The model under review builds one solid part; all positions refer to its coordinate system, in mm. Coordinates: 2 decimals unless noted, no trailing zeros. Loops run counter-clockwise (first coordinate to the right, second up) from the corner with the lowest first, then second, coordinate; pieces in that order, holes last. Notation, with made-up numbers: (15.5, 80.5) - (71.5, 80.5) arc R31 cw to (71.5, 118.5) - close; hole circle Ø1 at (16.5, -28.75). An arc over 180 degrees is marked (long way). Answer in a Markdown table with one row per item. Add a question column.
(1) We need section B-B on z = -37.5. Write out the cut boundary in (x, y), plus the area to 3 significant figures.
(2) We need section D-D on z = 7. Write out the cut boundary in (x, y), plus the area to 3 significant figures.
(3) We need section A-A on y = 5.5. Write out the cut boundary in (x, z), plus the area to 3 significant figures.
(4) We need section C-C on x = 8. Write out the cut boundary in (y, z), plus the area to 3 significant figures.
(5) For line 1 along X through (y, z) = (1.3, 39.5); line 2 along Y through (x, z) = (-46, 37.5); line 3 along X through (y, z) = (10.5, 38), list the stretches that pass through material, from the lowest coordinate up.
(6) For P1, Ø1, axis at x = -46, y = 7, coming from the -Z side; P2, Ø1.6, axis at x = -46.5, y = 6, coming from the +Z side; P3, Ø2, axis at y = 1, z = 0, coming from the -X side; P4, Ø4, axis at x = 27, y = 5.5, coming from the +Z side, all flat-tipped, find the tip position at first contact; note any pin that passes through.
from build123d import *

# Parameters (mm, degrees)
SKETCH1_W           = 95
SKETCH1_H           = 95
BOSS_EXTRUDE1_DEPTH = 2
SKETCH2_W           = 2
SKETCH2_H           = 6
BOSS_EXTRUDE2_DEPTH = 6
SKETCH3_R           = 3
BOSS_EXTRUDE3_DEPTH = 2
SKETCH6_R           = 3
BOSS_EXTRUDE5_DEPTH = 2
SKETCH8_R           = 1.3
CUT_EXTRUDE2_DEPTH  = 96
FILLET1_R           = 2
SKETCH10_W          = 25
SKETCH10_H          = 4
CUT_EXTRUDE3_DEPTH  = 5
SKETCH11_R          = 2.5
CUT_EXTRUDE4_DEPTH  = 2


with BuildPart() as part:
    # Sketch1 → Boss-Extrude1 (new body)
    with BuildSketch(Plane(origin=(0, 0, 0), x_dir=(1, 0, 0), z_dir=(0, 1, 0))):
        Rectangle(SKETCH1_W, SKETCH1_H)
    extrude(amount=BOSS_EXTRUDE1_DEPTH)

    # Sketch2 → Boss-Extrude2 (add)
    with BuildSketch(Plane(origin=(0, 2, 0), x_dir=(1, 0, 0), z_dir=(0, 1, 0))):
        with Locations((-46.5, -37.5)):
            Rectangle(SKETCH2_W, SKETCH2_H)
        with Locations((-46.5, 37.5)):
            Rectangle(SKETCH2_W, SKETCH2_H)
        with Locations((46.5, -37.5)):
            Rectangle(SKETCH2_W, SKETCH2_H)
        with Locations((46.5, 37.5)):
            Rectangle(SKETCH2_W, SKETCH2_H)
    extrude(amount=BOSS_EXTRUDE2_DEPTH)

    # Sketch3 → Boss-Extrude3 (add)
    with BuildSketch(Plane(origin=(-45.5, 0, 0), x_dir=(0, 0, -1), z_dir=(1, 0, 0))):
        with Locations((-37.5, 8)):
            Circle(SKETCH3_R)
        with Locations((37.5, 8)):
            Circle(SKETCH3_R)
    extrude(amount=-BOSS_EXTRUDE3_DEPTH)

    # Sketch6 → Boss-Extrude5 (add)
    with BuildSketch(Plane.ZY.offset(-45.5)):
        with Locations((-37.5, 8)):
            Circle(SKETCH6_R)
        with Locations((37.5, 8)):
            Circle(SKETCH6_R)
    extrude(amount=-BOSS_EXTRUDE5_DEPTH)

    # Sketch8 → Cut-Extrude2 (cut, through all)
    with BuildSketch(Plane.ZY.offset(47.5)):
        with Locations((-37.5, 8)):
            Circle(SKETCH8_R)
        with Locations((37.5, 8)):
            Circle(SKETCH8_R)
    extrude(amount=-CUT_EXTRUDE2_DEPTH, mode=Mode.SUBTRACT)

    # Fillet1
    fillet1_edges = [part.edges().sort_by_distance(p)[0] for p in [
        (-46.5, 2, 40.5),
        (-45.5, 2, 37.5),
        (-46.5, 2, 34.5),
        (-46.5, 2, -34.5),
        (-45.5, 2, -37.5),
        (-46.5, 2, -40.5),
        (46.5, 2, 34.5),
        (45.5, 2, 37.5),
        (46.5, 2, 40.5),
        (46.5, 2, -40.5),
        (45.5, 2, -37.5),
        (46.5, 2, -34.5),
    ]]
    fillet(fillet1_edges, radius=FILLET1_R)

    # Sketch10 → Cut-Extrude3 (cut)
    with BuildSketch(Plane.ZY.offset(47.5)):
        Rectangle(SKETCH10_W, SKETCH10_H)
    extrude(amount=-CUT_EXTRUDE3_DEPTH, mode=Mode.SUBTRACT)

    # Sketch11 → Cut-Extrude4 (cut)
    with BuildSketch(Plane(origin=(0, 2, 0), x_dir=(1, 0, 0), z_dir=(0, 1, 0))):
        with Locations((18, -39.5)):
            Circle(SKETCH11_R)
        with Locations((8, -39.5)):
            Circle(SKETCH11_R)
    extrude(amount=-CUT_EXTRUDE4_DEPTH, mode=Mode.SUBTRACT)


solid = part.part
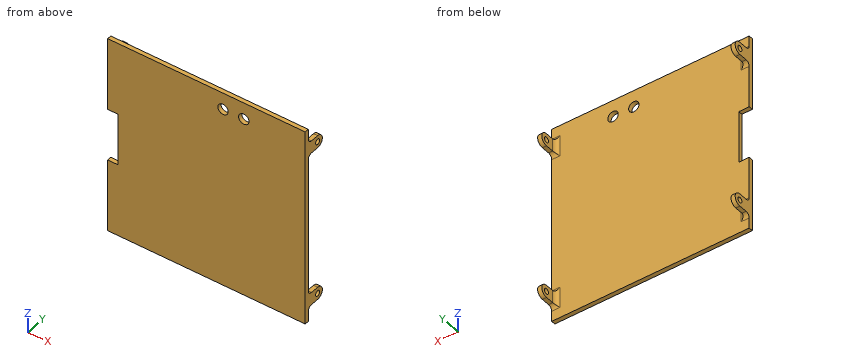
Outcome:
| question | item | result |
|---|---|---|
| 1 | outline | (-47.5, 0) - (47.5, 0) - (47.5, 6.7) - (45.5, 6.7) - (45.5, 4) arc R2 cw to (43.5, 2) - (-43.5, 2) arc R2 cw to (-45.5, 4) - (-45.5, 6.7) - (-47.5, 6.7) - close; (-47.5, 9.3) - (-45.5, 9.3) - (-45.5, 11) - (-47.5, 11) - close; (45.5, 9.3) - (47.5, 9.3) - (47.5, 11) - (45.5, 11) - close |
| 1 | area | 217 mm² |
| 2 | outline | (-42.5, 0) - (47.5, 0) - (47.5, 2) - (-42.5, 2) - close |
| 2 | area | 180 mm² |
| 3 | outline | (-47.5, -40.5) - (-45.5, -40.5) - (-45.5, -34.5) - (-47.5, -34.5) - close; (-47.5, 34.5) - (-45.5, 34.5) - (-45.5, 40.5) - (-47.5, 40.5) - close; (45.5, -40.5) - (47.5, -40.5) - (47.5, -34.5) - (45.5, -34.5) - close; (45.5, 34.5) - (47.5, 34.5) - (47.5, 40.5) - (45.5, 40.5) - close |
| 3 | area | 48.0 mm² |
| 4 | outline | (0, -47.5) - (2, -47.5) - (2, 37) - (0, 37) - close; (0, 42) - (2, 42) - (2, 47.5) - (0, 47.5) - close |
| 4 | area | 180 mm² |
| 5 | line 1 | -47.5 to 5.5, 10.5 to 15.5, 20.5 to 47.5 |
| 5 | line 2 | 0 to 6.7, 9.3 to 11 |
| 5 | line 3 | -47.5 to -45.5, 45.5 to 47.5 |
| 6 | P1 | z = -40.5 |
| 6 | P2 | z = 40.5 |
| 6 | P3 | x = -42.5 |
| 6 | P4 | through |
